```python
from build123d import *

# Parameters (mm, degrees)
BOSS_EXTRUDE1_DEPTH = 40


with BuildPart() as part:
    # Sketch1 → Boss-Extrude1 (new, symmetric)
    with BuildSketch(Plane.YZ):
        Polygon((-30, 30), (-15, 30), (-2.5, 10), (-2.5, 5), (2.5, 5), (2.5, 10), (15, 30), (30, 30), (30, 5), (25, 5), (25, -5), (30, -5), (30, -30), (15, -30), (2.5, -10), (2.5, -5), (-2.5, -5), (-2.5, -10), (-15, -30), (-30, -30), (-30, -5), (-25, -5), (-25, 5), (-30, 5), align=None)
    extrude(amount=BOSS_EXTRUDE1_DEPTH, both=True)


solid = part.part
```
Could you check a few things on this model? Use its own coordinates, in mm. A direction names the side the tool comes from. Round coordinates to 2 decimals unless told otherwise and drop trailing zeros. Loops run counter-clockwise (first coordinate to the right, second up) from the corner with the lowest first, then second, coordinate; pieces in that order, holes last. Notation, with made-up numbers: (29, 34.5) - (58, 34.5) arc R28 ccw to (58, 69.5) - close; hole circle Ø7 at (-35, 18.5). An arc over 180 degrees is marked (long way). Use CSV: the item, a comma, the result in double quotes.
Item 1: If we section it at A-A on z = 14: List the corners of the cut face in (x, y) for me, then the cut area to 3 significant figures.
Here are the results:
outline,"(-40, -30) - (40, -30) - (40, -5) - (-40, -5) - close; (-40, 5) - (40, 5) - (40, 30) - (-40, 30) - close"
area,"4,000 mm²"
Item 2: I need wall thicknesses on L1, parallel to Y at x = -27.5, z = -10; L2, parallel to Z at x = 20, y = 1.5; L3, parallel to Y at x = 29, z = 16. Which ranges of each line are inside material? Lowest first, please. Write a range as [from, to].
Here are the results:
L1,"y = [-30, -2.5], [2.5, 30]"
L2,"z = [-5, 5]"
L3,"y = [-30, -6.25], [6.25, 30]"
Item 3: Will these pins go through, and if not, where does the flat tip stop? pin 1 (2.5 mm diameter, centred on x = 17, y = 0.5, fed in from -Z); pin 2 (3 mm diameter, centred on x = 6, z = 0, fed in from -Y); pin 3 (1.5 mm diameter, centred on x = 4, y = -0.5, fed in from +Z); pin 4 (11 mm diameter, centred on x = -0.5, z = -1.5, fed in from +Y).
Here are the results:
pin 1,"stops at z = -5"
pin 2,"stops at y = -25"
pin 3,"stops at z = 5"
pin 4,"stops at y = 30"
Item 4: For faces 5 (the flat face through (0.56, 8.663, 19.86)), 6 (the flat face through (0.56, 8.837, -20.14)), 7 (the flat face through (1, 28, 5)), 8 (the flat face through (1, -28, -5)), which set-ups out of +Z, -Z, +X, -X, +Y, -Y let a thin tool reach every point of the face, with its end or its side?
Here are the results:
face 5,"+Z, +X, -X"
face 6,"-Z, +X, -X"
face 7,"+X, -X, +Y"
face 8,"+X, -X, -Y"
Item 5: If we section it at C-C on z = -7: List the corners of the cut face in (x, y) for me, then the cut area to 3 significant figures.
Here are the results:
outline,"(-40, -30) - (40, -30) - (40, -2.5) - (-40, -2.5) - close; (-40, 2.5) - (40, 2.5) - (40, 30) - (-40, 30) - close"
area,"4,400 mm²"
Item 6: If we section it at B-B on x = -16.5: List the corners of the cut face in (y, z) for me.
Here are the results:
outline,"(-30, -30) - (-15, -30) - (-2.5, -10) - (-2.5, -5) - (2.5, -5) - (2.5, -10) - (15, -30) - (30, -30) - (30, -5) - (25, -5) - (25, 5) - (30, 5) - (30, 30) - (15, 30) - (2.5, 10) - (2.5, 5) - (-2.5, 5) - (-2.5, 10) - (-15, 30) - (-30, 30) - (-30, 5) - (-25, 5) - (-25, -5) - (-30, -5) - close"
Item 7: If we section it at D-D on y = 11: List the corners of the cut face in (x, z) for me, then the cut area to 3 significant figures.
Here are the results:
outline,"(-40, -23.6) - (40, -23.6) - (40, 23.6) - (-40, 23.6) - close"
area,"3,780 mm²"
Item 8: If we mould it in two halves opening along Z, with no side actions, what happens to faces 1 (the flat face through (1, -25, 0)), 2 (the flat face through (1, 25, 0)), 3 (the flat face through (0.56, -8.663, -19.86)), 4 (the flat face through (-40, 0, 0))? For each: pulls with the +Z half, pulls with the -Z half, needs draft (parallel to the pull), parting line crosses it, or undercut.
Here are the results:
face 1,"undercut"
face 2,"undercut"
face 3,"pulls with the -Z half"
face 4,"needs draft"
